from build123d import *

# Parameters (mm, degrees)
F1_DEPTH = 0.79375
F3_D     = 4


with BuildPart() as f1:
    # F0 (on Right) → F1 (new body, symmetric)
    with BuildSketch(Plane.YZ):
        with BuildLine():
            ThreePointArc((3.175, 12.7), (-1.315128, 10.840128), (-3.175, 6.35))
            Line((-3.175, 6.35), (-3.175, -6.35))
            ThreePointArc((-3.175, -6.35), (-1.315128, -10.840128), (3.175, -12.7))
            ThreePointArc((3.175, -12.7), (6.35, -9.525), (3.175, -6.35))
            Line((3.175, -6.35), (3.175, 6.35))
            ThreePointArc((3.175, 6.35), (6.35, 9.525), (3.175, 12.7))
        make_face()
    extrude(amount=F1_DEPTH, both=True)

    # F3 (through all)
    with Locations(Plane.YZ.offset(0.79375)):
        with Locations((3.175, 9.525), (3.175, -9.525)):
            Hole(F3_D / 2)


solid = f1.part
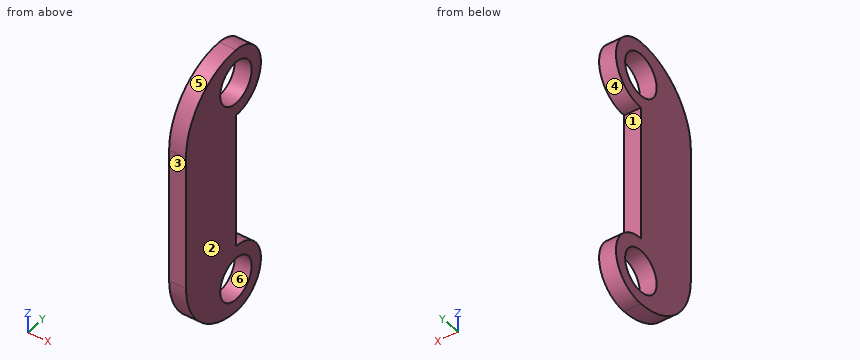
Design review of the part built by this model. Coordinates are the model's own, in mm. Face numbers are marked on the shaded views. A direction names the side the tool comes from. Round coordinates to 2 decimals unless told otherwise and drop trailing zeros. Order: outer loops, then holes, each group sorted by start corner. A loop starts at its lowest first (then second) coordinate and runs counter-clockwise, first axis right, second up. Notation, with made-up numbers: M -17,46 L 36,46 A33 ccw 36,81 Z; hole C 60,18.25 d10. An arc over 180 degrees is marked long. Answer as CSV lines item,"result". Start each with the question number.
1) The part is to be moulded in two halves that separate along Z. For the marked faces 3, 4, 5 and 6, say which applies: +Z half, -Z half, draft (parallel to the pull), parting line (faces both ways), or undercut.
2) Add section D-D (y = 5.75). Give the boundary of the cut face in (x, z).
3) Add section B-B (x = -0.3). Give the boundary of the cut face in (y, z) (3 decimals).
4) Add section A-A (z = 10.75). Give the boundary of the cut face in (x, y), then the cut area to 3 significant figures.
5) Tool access review of the marked faces 1 and 2: name each direction out of +Z, -Z, +X, -X, +Y, -Y from which nothing blocks a thin tool from reaching the whole face with its end or side.
6) Add section C-C (y = 4). Give the boundary of the cut face in (x, z).
7) Wall thickness on line 1 along Z through (x, y) = (-0.4, 3.25); line 2 along Z through (x, y) = (-0.3, 5); line 3 along Z through (x, y) = (0.1, 1.5): over which ranges is each line inside the solid? List them lowest first. Write a range as [from, to].
Resolved:
1,face 3,"draft"
1,face 4,"undercut"
1,face 5,"+Z half"
1,face 6,"undercut"
2,outline,"M -0.79,-11.38 L 0.79,-11.38 L 0.79,-7.67 L -0.79,-7.67 Z; M -0.79,7.67 L 0.79,7.67 L 0.79,11.38 L -0.79,11.38 Z"
3,outline,"M -3.175,-6.35 A6.35 ccw 3.175,-12.7 A3.175 ccw 3.175,-6.35 L 3.175,6.35 A3.175 ccw 3.175,12.7 A6.35 ccw -3.175,6.35 Z; hole C 3.175,-9.525 d4; hole C 3.175,9.525 d4"
4,outline,"M -0.79,-1.4 L 0.79,-1.4 L 0.79,1.59 L -0.79,1.59 Z; M -0.79,4.76 L 0.79,4.76 L 0.79,6.1 L -0.79,6.1 Z"
4,area,"6.90 mm^2"
5,face 1,"+X, -X, +Y"
5,face 2,"+Z, -Z, +X, +Y, -Y"
6,outline,"M -0.79,-12.59 L 0.79,-12.59 L 0.79,-11.35 L -0.79,-11.35 Z; M -0.79,-7.7 L 0.79,-7.7 L 0.79,-6.46 L -0.79,-6.46 Z; M -0.79,6.46 L 0.79,6.46 L 0.79,7.7 L -0.79,7.7 Z; M -0.79,11.35 L 0.79,11.35 L 0.79,12.59 L -0.79,12.59 Z"
7,line 1,"[-12.7, -11.52], [-7.53, -6.35], [6.35, 7.53], [11.52, 12.7]"
7,line 2,"[-12.12, -10.34], [-8.71, -6.93], [6.93, 8.71], [10.34, 12.12]"
7,line 3,"[-12.48, -10.62], [-8.43, 8.43], [10.62, 12.48]"
